```python
from build123d import *

# Parameters (mm, degrees)
BOSS_EXTRUDE3_DEPTH = 5
SKETCH2_W           = 5
SKETCH2_H           = 16
CUT_EXTRUDE1_DEPTH  = 140.606590102
SKETCH3_R           = 3
CUT_EXTRUDE2_DEPTH  = 140.606590102


with BuildPart() as part:
    # Sketch1 → Boss-Extrude3 (new body)
    with BuildSketch(Plane.XY):
        Polygon((0, 0), (38.61949762, 0), (38.61949762, -31), (48.11949762, -31), (48.11949762, -41), (64.11949762, -41), (64.11949762, -31), (73.61949762, -31), (73.61949762, 0), (117, 0), (117, 35), (73.61949762, 35), (73.61949762, 66), (64.11949762, 66), (64.11949762, 76), (48.11949762, 76), (48.11949762, 66), (38.61949762, 66), (38.61949762, 35), (0, 35), align=None)
    extrude(amount=BOSS_EXTRUDE3_DEPTH)

    # Sketch2 → Cut-Extrude1 (cut, through all)
    with BuildSketch(Plane.XY.offset(5)):
        with Locations((7.5, 17.5)):
            Rectangle(SKETCH2_W, SKETCH2_H)
        with Locations((109.5, 17.5)):
            Rectangle(SKETCH2_W, SKETCH2_H)
    extrude(amount=-CUT_EXTRUDE1_DEPTH, mode=Mode.SUBTRACT)

    # Sketch3 → Cut-Extrude2 (cut, through all)
    with BuildSketch(Plane.XY.offset(5)):
        with Locations((56.11949762, 17.5)):
            Circle(SKETCH3_R)
    extrude(amount=-CUT_EXTRUDE2_DEPTH, mode=Mode.SUBTRACT)


solid = part.part
```
CAD build for the part. Positions are in the model's coordinates, mm. A direction names the side the tool comes from. Round coordinates to 2 decimals unless told otherwise and drop trailing zeros. Loops run counter-clockwise (first coordinate to the right, second up) from the corner with the lowest first, then second, coordinate; pieces in that order, holes last. Notation, with made-up numbers: (56.5, 88.5) - (110.5, 88.5) arc R30 cw to (110.5, 115.5) - close; hole circle Ø7 at (23.5, -4). An arc over 180 degrees is marked (long way). Return JSON: item names as keys, results as strings. Group by question number.
Q1. Band-saw the part on C-C on y = 67.5. Give the cut face in (x, z).
Q2. Flat gauge pins, fed straight in: pin 1 Ø2.5 at (y, z) = (51, 3.5) entering from -X; pin 2 Ø1.5 at (x, z) = (68, 1.5) entering from +Y; pin 3 Ø2.5 at (y, z) = (69, 1.5) entering from +X. Where does each tip first touch, or does it go through?
Q3. Band-saw the part on B-B on z = 1.8. Give the number of separate pieces and of enclosed holes in the cut face, plus the area to 3 significant figures.
Q4. Tool access for faces 5 (the face through (64.119, -36, 2)), 6 (the face through (19, 0, 2)), 7 (the face through (107, 17, 3)), 8 (the face through (64.119, 71, 2)): list every direction of +Z, -Z, +X, -X, +Y, -Y with a clear straight run to the whole face (end or side of a thin tool).
Q5. Band-saw the part on D-D on x = 105. Give the cut face in (y, z), plus the area to 3 significant figures.
Q6. Band-saw the part on A-A on y = 17.5. Give the cut face in (x, z), plus the area to 3 significant figures.
Q7. Drill centre lines: line 1 along Y through (x, z) = (104, 1.75); line 2 along X through (y, z) = (-23.5, 2); line 3 along Y through (x, z) = (48, 2.8). Where is each one in solid material? Low to high. Write a range as [from, to].
Q8. Two-plate mould, pull along X, no slides. Class faces 1 (the face through (7, 9.5, 3)), 2 (the face through (43, 66, 2)), 3 (the face through (73.619, 50, 2)), 4 (the face through (48.119, -36, 2)): +X half, -X half, draft (parallel to the pull), parting line (faces both ways), or undercut.
Solutions:
{
 "1": {"outline": "(48.12, 0) - (64.12, 0) - (64.12, 5) - (48.12, 5) - close"},
 "2": {"pin 1": "stops at x = 38.62", "pin 2": "stops at y = 66", "pin 3": "stops at x = 64.12"},
 "3": {"separate pieces": "1", "enclosed holes": "3", "area": "6,400 mm^2"},
 "4": {"face 5": "+Z, -Z, +X, -Y", "face 6": "+Z, -Z, -X, -Y", "face 7": "+Z, -Z", "face 8": "+Z, -Z, +X, +Y"},
 "5": {"outline": "(0, 0) - (35, 0) - (35, 5) - (0, 5) - close", "area": "175 mm^2"},
 "6": {"outline": "(0, 0) - (5, 0) - (5, 5) - (0, 5) - close; (10, 0) - (53.12, 0) - (53.12, 5) - (10, 5) - close; (59.12, 0) - (107, 0) - (107, 5) - (59.12, 5) - close; (112, 0) - (117, 0) - (117, 5) - (112, 5) - close", "area": "505 mm^2"},
 "7": {"line 1": "y = [0, 35]", "line 2": "x = [38.62, 73.62]", "line 3": "y = [-31, 66]"},
 "8": {"face 1": "undercut", "face 2": "draft", "face 3": "+X half", "face 4": "-X half"}
}
